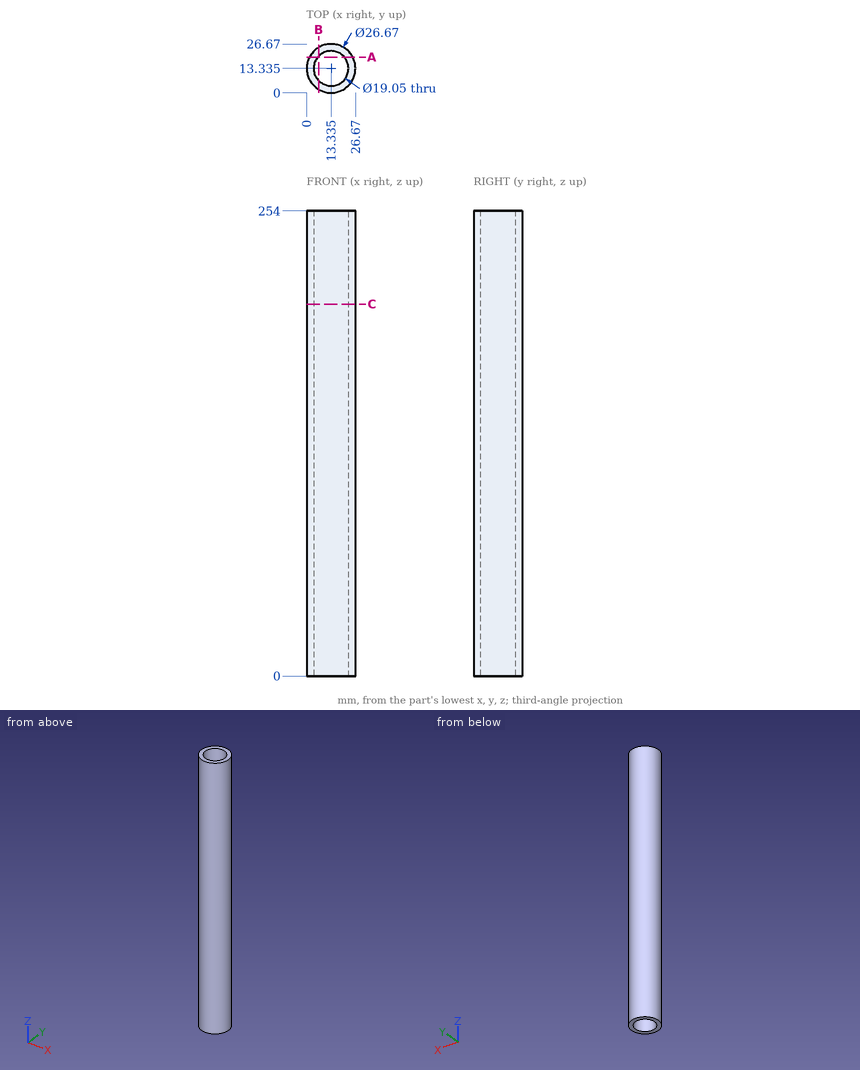
Geometry: see drawing. Coordinates: mm, zero at the bounding-box minimum. Coordinates: 2 decimals unless noted, no trailing zeros. Loops run counter-clockwise (first coordinate to the right, second up) from the corner with the lowest first, then second, coordinate; pieces in that order, holes last.
Q1. Cut plane C-C (z = 203). Output: boundary loops of the cut face in (x, y) (3 decimals).
Q2. Cut plane A-A (y = 19.5). Output: boundary loops of the cut face in (x, z).
Q3. Material intervals for line 1 (Y direction, x = 14.25, z = 122); line 2 (Y direction, x = 12, z = 190.5); line 3 (X direction, y = 10.5, z = 50), sorted ascending.
Q4. Contact query for flat-ended pins moving along their axis: pin 1 (1 mm diameter, centred on y = 12, z = 119.5, fed in from -X); pin 2 (12 mm diameter, centred on x = 6, z = 65.5, fed in from -Y); pin 3 (2 mm diameter, centred on y = 10.5, z = 211, fed in from +X). Output: stop coordinate, or through.
Q5. Cut plane B-B (x = 6.5). Output: boundary loops of the cut face in (y, z), then the cut area to 3 significant figures.
Working result:
1. outline: circle Ø26.67 at (13.335, 13.335); hole circle Ø19.05 at (13.335, 13.335)
2. outline: (1.51, 0) - (6.07, 0) - (6.07, 254) - (1.51, 254) - close; (20.6, 0) - (25.16, 0) - (25.16, 254) - (20.6, 254) - close
3. line 1: y = 0.03 to 3.85, 22.82 to 26.64
3. line 2: y = 0.07 to 3.9, 22.77 to 26.6
3. line 3: x = 0.3 to 4.24, 22.43 to 26.37
4. pin 1: stops at x = 0.03
4. pin 2: stops at y = 0.07
4. pin 3: stops at x = 26.54
5. outline: (1.88, 0) - (6.7, 0) - (6.7, 254) - (1.88, 254) - close; (19.97, 0) - (24.79, 0) - (24.79, 254) - (19.97, 254) - close
5. area: 2,450 mm2
